Geometry: final body of the model. Coordinates: model frame, mm. A direction names the side the tool comes from. Give positions to 0.01 mm unless a question says otherwise; leave off trailing zeros. Write each loop counter-clockwise with the first axis right and the second up, starting at its lowest first coordinate (ties: lowest second). Pieces come first, ordered by that corner, then holes. Notation, with made-up numbers: (44, 49.5) -> (82, 49.5) arc R30 ccw to (82, 74.5) -> close; hole circle Ø6 at (50, -28.5). An arc over 180 degrees is marked (long way). Answer in a Markdown table with one row per item. Add a question column.
Item 1: Access query for faces 1 (the cylindrical face through (-9, 0.3, 21.4)), 2 (the cylindrical face through (-96.97, -0.99, 15.96)), 3 (the flat face through (-3.5, 0, 7.7)). Directions: +Z, -Z, +X, -X, +Y, -Y. A direction counts if a zero-diameter tool reaches every point of the face in a straight line with its end or side. Return the directions, or none.
Item 2: First-contact query: P1, Ø1, axis at x = -78, y = -0.5, coming from the -Z side; P2, Ø0.8, axis at x = -80, y = 0.5, coming from the +Z side; P3, Ø0.5, axis at y = 1, z = 5.5, coming from the +X side. Flat tips, straight axial feed; report the tip coordinate or a pass-through.
Item 3: Section query B-B on z = 17.5. State how many separate pieces and enclosed holes the cut face has, plus the area to 3 significant figures.
Item 4: Material intervals for probe 1 along Z at (x, y) = (-54.5, 0.75); probe 2 along Y at (x, z) = (-86, 26); probe 3 along Z at (x, y) = (-5.6, -0.4), sorted ascending. Write a range as from..to.
Item 5: Section query A-A on x = -42. Output: boundary loops of the cut face in (y, z), plus the area to 3 significant figures.
Item 6: Section query C-C on x = -199. Output: boundary loops of the cut face in (y, z), plus the area to 3 significant figures.
Item 7: Section query D-D on z = -35. Output: boundary loops of the cut face in (x, y).
Item 8: Draft query along X for faces 4 (the cylindrical face through (-59.18, -0.39, 18.79)), 5 (the cylindrical face through (-192, -1, 10.8)), 6 (the flat face through (-150, -2, 6)). Return one class per face: +X half, -X half, draft (parallel to the pull), parting line (faces both ways), or undercut.
```python
from build123d import *

# Parameters (mm, degrees)
SKETCH074_R      = 1.8
SKETCH074_R_2    = 6.3
PAD004_DEPTH     = 2
SKETCH091_R      = 7.3
POCKET001_DEPTH  = 1.2
SKETCH092_W      = 82.8
SKETCH092_H      = 36
SKETCH092_R      = 1.8
PAD005_DEPTH     = 1.6
CHAMFER001_SIZE2 = 3.4
CHAMFER001_SIZE  = 2.4
POCKET002_DEPTH  = 1.6
CHAMFER002_SIZE  = 1


with BuildPart() as part:
    # Sketch074 → Pad004 (new body)
    with BuildSketch(Plane.XZ):
        with BuildLine():
            Line((-82.8, 3.2), (0, 3.2))
            Line((0, 3.2), (0, 39.2))
            Line((-195.886839, 39.2), (0, 39.2))
            Line((-202.764796, 20.302968), (-195.886839, 39.2))
            ThreePointArc((-192.175575, -3.18451), (-192.085048, 10.987093), (-202.764796, 20.302968))
            Line((-192.175575, -3.18451), (-215.419579, -53.031439))
            ThreePointArc((-215.419579, -53.031439), (-218.578907, -66.677212), (-215.93199, -80.431568))
            Line((-215.93199, -80.431568), (-176.68528, -80.431568))
            Line((-147.645309, 8.944272), (-176.68528, -80.431568))
            ThreePointArc((-132.428405, 20), (-141.832969, 16.944272), (-147.645309, 8.944272))
            Line((-132.428405, 20), (-107.6, 20))
            ThreePointArc((-91.751972, 6.2), (-97.09286, 16.066483), (-107.6, 20))
            Line((-82.8, 6.2), (-91.751972, 6.2))
            Line((-82.8, 3.2), (-82.8, 6.2))
        make_face()
        with Locations((-213.443268, -76.831568)):
            Circle(SKETCH074_R, mode=Mode.SUBTRACT)
        with Locations((-179.304663, -76.831568)):
            Circle(SKETCH074_R, mode=Mode.SUBTRACT)
        with Locations((-184.079668, 34.8)):
            Circle(SKETCH074_R, mode=Mode.SUBTRACT)
        with Locations((-78.51, 34.8)):
            Circle(SKETCH074_R, mode=Mode.SUBTRACT)
        with Locations((-78.51, 7.6)):
            Circle(SKETCH074_R, mode=Mode.SUBTRACT)
        with Locations((-5.6, 34.8)):
            Circle(SKETCH074_R, mode=Mode.SUBTRACT)
        with Locations((-5.6, 7.6)):
            Circle(SKETCH074_R, mode=Mode.SUBTRACT)
        with Locations((-19, 21.2)):
            Circle(SKETCH074_R_2, mode=Mode.SUBTRACT)
        with Locations((-42, 21.2)):
            Circle(SKETCH074_R_2, mode=Mode.SUBTRACT)
        with Locations((-65, 21.2)):
            Circle(SKETCH074_R_2, mode=Mode.SUBTRACT)
        Polygon((-189.938695, 31.567195), (-192.332836, 24.989347), (-196.467483, 26.494236), (-194.073342, 33.072084), (-193.885404, 33.00368), (-190.126633, 31.635599), align=None, mode=Mode.SUBTRACT)
    extrude(amount=PAD004_DEPTH)

    # Sketch091 (on Face29 of Pad004) → Pocket001 (cut)
    with BuildSketch(Plane.XZ.offset(2)):
        with Locations((-65, 21.2)):
            Circle(SKETCH091_R)
        with Locations((-42, 21.2)):
            Circle(SKETCH091_R)
        with Locations((-19, 21.2)):
            Circle(SKETCH091_R)
    extrude(amount=-POCKET001_DEPTH, mode=Mode.SUBTRACT)

    # Sketch092 (on Face4 of Pocket001) → Pad005 (join)
    with BuildSketch(Plane(origin=(0, 0, 0), x_dir=(1, 0, 0), z_dir=(0, 1, 0))):
        with Locations((-41.4, -21.2)):
            Rectangle(SKETCH092_W, SKETCH092_H)
        with Locations((-5.6, -34.8)):
            Circle(SKETCH092_R, mode=Mode.SUBTRACT)
        with Locations((-5.6, -7.6)):
            Circle(SKETCH092_R, mode=Mode.SUBTRACT)
        with Locations((-78.51, -34.8)):
            Circle(SKETCH092_R, mode=Mode.SUBTRACT)
        with Locations((-78.51, -7.6)):
            Circle(SKETCH092_R, mode=Mode.SUBTRACT)
        with BuildLine():
            ThreePointArc((-19, -31.2), (-9, -21.2), (-19, -11.2))
            Line((-19, -11.2), (-65, -11.2))
            ThreePointArc((-65, -11.2), (-75, -21.2), (-65, -31.2))
            Line((-19, -31.2), (-65, -31.2))
        make_face(mode=Mode.SUBTRACT)
    extrude(amount=PAD005_DEPTH)

    # Chamfer001
    chamfer001_edges = [part.edges().sort_by_distance(p)[0] for p in [
        (0, 1.6, 21.2),
        (-41.4, 1.6, 3.2),
        (-82.8, 1.6, 21.2),
    ]]
    chamfer001_side = part.faces().sort_by_distance((-41.4, 1.6, 4.102875))[0]
    chamfer(chamfer001_edges, length=CHAMFER001_SIZE, length2=CHAMFER001_SIZE2, reference=chamfer001_side)

    # Sketch093 (on Face1 of Chamfer001) → Pocket002 (cut)
    with BuildSketch(Plane(origin=(0, 1.6, 0), x_dir=(1, 0, 0), z_dir=(0, 1, 0))):
        with BuildLine():
            ThreePointArc((-5.6, -31.3), (-8.074874, -32.325126), (-9.1, -34.8))
            Line((-9.1, -39.2), (-9.1, -34.8))
            Line((0, -39.2), (-9.1, -39.2))
            Line((0, -39.2), (0, -31.3))
            Line((0, -31.3), (-5.6, -31.3))
        make_face()
        with BuildLine():
            ThreePointArc((-75.01, -34.8), (-76.035126, -32.325126), (-78.51, -31.3))
            Line((-82.8, -31.3), (-78.51, -31.3))
            Line((-82.8, -39.2), (-82.8, -31.3))
            Line((-82.8, -39.2), (-75.01, -39.2))
            Line((-75.01, -39.2), (-75.01, -34.8))
        make_face()
        with BuildLine():
            ThreePointArc((-9.1, -7.6), (-8.074874, -10.074874), (-5.6, -11.1))
            Line((0, -11.1), (-5.6, -11.1))
            Line((0, -3.2), (0, -11.1))
            Line((0, -3.2), (-9.1, -3.2))
            Line((-9.1, -3.2), (-9.1, -7.6))
        make_face()
        with BuildLine():
            ThreePointArc((-78.51, -11.1), (-76.035126, -10.074874), (-75.01, -7.6))
            Line((-75.01, -3.2), (-75.01, -7.6))
            Line((-82.8, -3.2), (-75.01, -3.2))
            Line((-82.8, -3.2), (-82.8, -11.1))
            Line((-82.8, -11.1), (-78.51, -11.1))
        make_face()
    extrude(amount=-POCKET002_DEPTH, mode=Mode.SUBTRACT)

    # Chamfer002
    chamfer002_edges = [part.edges().sort_by_distance(p)[0] for p in [
        (-42, 1.6, 31.2),
        (-9, 1.6, 21.2),
        (-42, 1.6, 11.2),
        (-75, 1.6, 21.2),
    ]]
    chamfer(chamfer002_edges, length=CHAMFER002_SIZE)


solid = part.part
```
Findings below:
| question | item | result |
|---|---|---|
| 1 | face 1 | +Y |
| 1 | face 2 | -Z, +Y, -Y |
| 1 | face 3 | -Z, +X, +Y |
| 2 | P1 | stops at z = 3.76 |
| 2 | P2 | stops at z = 31.3 |
| 2 | P3 | stops at x = -9.1 |
| 3 | separate pieces | 5 |
| 3 | enclosed holes | 0 |
| 3 | area | 262 mm^2 |
| 4 | probe 1 | z = 5..11.05, 31.35..39.2 |
| 4 | probe 2 | y = -2..0 |
| 4 | probe 3 | z = 4.19..5.8, 9.4..33, 36.6..39.2 |
| 5 | outline | (-2, 3.2) -> (-1.8, 3.2) -> (1.6, 5.6) -> (1.6, 10.2) -> (0.6, 11.2) -> (0, 11.2) -> (0, 14.9) -> (-0.8, 14.9) -> (-0.8, 13.9) -> (-2, 13.9) -> close; (-2, 28.5) -> (-0.8, 28.5) -> (-0.8, 27.5) -> (0, 27.5) -> (0, 31.2) -> (0.6, 31.2) -> (1.6, 32.2) -> (1.6, 39.2) -> (-2, 39.2) -> close |
| 5 | area | 64.9 mm^2 |
| 6 | outline | (-2, -80.43) -> (0, -80.43) -> (0, -17.82) -> (-2, -17.82) -> close; (-2, 18.67) -> (0, 18.67) -> (0, 30.65) -> (-2, 30.65) -> close |
| 6 | area | 149 mm^2 |
| 7 | outline | (-207.01, -2) -> (-161.92, -2) -> (-161.92, 0) -> (-207.01, 0) -> close |
| 8 | face 4 | undercut |
| 8 | face 5 | -X half |
| 8 | face 6 | draft |
